Could you check a few things on this model? Use its own coordinates, in mm. A direction names the side the tool comes from. Give positions to 0.01 mm unless a question says otherwise; leave off trailing zeros. Loops run counter-clockwise (first coordinate to the right, second up) from the corner with the lowest first, then second, coordinate; pieces in that order, holes last.
1. I need wall thicknesses on line 1 along X through (y, z) = (-6.5, 2.5); line 2 along X through (y, z) = (-9, 28.5); line 3 along Y through (x, z) = (-15, 22). Which ranges of each line are inside material? Lowest first, please.
2. Imagine slicing it at A-A (z = 20.5). List the corners of the cut face in (x, y) for me.
3. For faces 1 (the cylindrical face through (1.382, -21.456, 21.902)), 2 (the flat face through (19, 0, 12)), which set-ups out of +Z, -Z, +X, -X, +Y, -Y let a thin tool reach every point of the face, with its end or its side?
4. Thinking about a two-plate mould opening in X: for faces 3 (the cylindrical face through (2, -30.935, 2.268)), 4 (the cylindrical face through (0.864, -13.472, 15.196)), 5 (the flat face through (0, -15, 30)), which applies, +X half, -X half, draft (parallel to the pull), parting line (faces both ways), or undercut?
5. For P1, Ø4, axis at x = 7.5, y = -25, coming from the +Z side; P2, Ø3, axis at x = -11, y = -20, coming from the +Z side; P3, Ø10, axis at x = -16.5, z = 13, coming from the -Y side, each with a flat end and sliding along its axis, tell me the tip position at first contact or that it passes through.
```python
from build123d import *

# Parameters (mm, degrees)
REVOLUTION_ANGLE = -175
FILLET_R         = 1


with BuildPart() as part:
    # Sketch → Revolution (revolve)
    with BuildSketch(Plane.XZ):
        Polygon((13.5, 0), (13.5, 30), (21.5, 30), (21.5, 15), (31, 5), (31, 0), align=None)
    revolve(axis=Axis((0, 0, 0), (0, 0, 1)), revolution_arc=REVOLUTION_ANGLE)

    # Fillet
    fillet_edges = [part.edges().sort_by_distance(p)[0] for p in [
        (0.588862, -13.487151, 0),
        (-13.448628, -1.176603, 15),
        (13.5, 0, 15),
        (0.588862, -13.487151, 30),
        (0.937817, -21.479537, 30),
        (1.352201, -30.970495, 5),
        (22.25, 0, 0),
        (-22.165332, -1.939215, 0),
        (17.5, 0, 30),
        (-17.433407, -1.525225, 30),
        (31, 0, 2.5),
        (26.25, 0, 10),
        (21.5, 0, 22.5),
        (-30.882036, -2.701828, 2.5),
        (-26.150111, -2.287838, 10),
        (-21.418186, -1.873848, 22.5),
    ]]
    fillet(fillet_edges, radius=FILLET_R)


solid = part.part
```
Derived:
1. line 1: x = -30.31 to -11.83, 11.83 to 30.31
1. line 2: x = -19.53 to -10.06, 10.06 to 19.53
1. line 3: y = -15.4 to -1.31
2. outline: (-21.3, -2.92) arc R21.5 ccw to (21.47, -1.05) arc R1 ccw to (20.48, 0) - (14.47, 0) arc R1 ccw to (13.47, -0.93) arc R13.5 cw to (-13.34, -2.1) arc R1 ccw to (-14.41, -1.26) - (-20.4, -1.78) arc R1 ccw to start
3. face 1: +Z, -Y
3. face 2: +Z, -Z, +X, -X, +Y
4. face 3: parting line
4. face 4: undercut
4. face 5: draft
5. P1: stops at z = 12.26
5. P2: stops at z = 29.56
5. P3: stops at y = -23.69
